```python
from build123d import *

# Parameters (mm, degrees)
SKETCH1_R               = 30
BOSS_EXTRUDE1_DEPTH     = 5
SKETCH2_R               = 20
SKETCH2_R_2             = 15
BOSS_EXTRUDE2_DEPTH     = 14.5
CUT_EXTRUDE1_START      = -20
SKETCH3_R               = 15
CUT_EXTRUDE1_DEPTH      = 20
CUT_EXTRUDE3_DEPTH      = 47.693147249
CUT_EXTRUDE3_DEPTH_BACK = 47.693147249
SKETCH5_R               = 2.5
SKETCH6_R               = 1.55
CUT_EXTRUDE4_DEPTH      = 10


with BuildPart() as part:
    # Sketch1 → Boss-Extrude1 (new body)
    with BuildSketch(Plane.XY):
        Circle(SKETCH1_R)
    extrude(amount=BOSS_EXTRUDE1_DEPTH)

    # Sketch2 → Boss-Extrude2 (add)
    with BuildSketch(Plane.XY.offset(5)):
        with Locations(Location((0, 0, 0), (0, 0, 180))):
            Circle(SKETCH2_R)
        with Locations(Location((0, 0, 0), (0, 0, 180))):
            Circle(SKETCH2_R_2, mode=Mode.SUBTRACT)
    extrude(amount=BOSS_EXTRUDE2_DEPTH)

    # Sketch3 → Cut-Extrude1 (cut)
    with BuildSketch(Plane.XY.offset(5).offset(CUT_EXTRUDE1_START)):
        with Locations(Location((0, 0, 0), (0, 0, 180))):
            Circle(SKETCH3_R)
    extrude(amount=CUT_EXTRUDE1_DEPTH, mode=Mode.SUBTRACT)

    # Sketch5 → Cut-Extrude3 (cut, two sides: drawn at the far end of the back side and taken through both)
    with BuildSketch(Plane(origin=(0, 0, 0), x_dir=(1, 0, 0), z_dir=(0, 1, 0)).offset(-CUT_EXTRUDE3_DEPTH_BACK)):
        with Locations(Location((0, -12.5, 0), (0, 0, 270))):
            Circle(SKETCH5_R)
    extrude(amount=CUT_EXTRUDE3_DEPTH + CUT_EXTRUDE3_DEPTH_BACK, mode=Mode.SUBTRACT)

    # Sketch6 → Cut-Extrude4 (cut)
    with BuildSketch(Plane.XY.offset(5)):
        with Locations((0, 25)):
            Circle(SKETCH6_R)
        with Locations((21.650635095, 12.5)):
            Circle(SKETCH6_R)
        with Locations((21.650635095, -12.5)):
            Circle(SKETCH6_R)
        with Locations((0, -25)):
            Circle(SKETCH6_R)
        with Locations((-21.650635095, -12.5)):
            Circle(SKETCH6_R)
        with Locations((-21.650635095, 12.5)):
            Circle(SKETCH6_R)
    extrude(amount=-CUT_EXTRUDE4_DEPTH, mode=Mode.SUBTRACT)


solid = part.part
```
Read the model definition and answer for the solid it produces. Units are mm, in the model's axes. A direction names the side the tool comes from. Coordinates: 2 decimals unless noted, no trailing zeros. Order: outer loops, then holes, each group sorted by start corner. A loop starts at its lowest first (then second) coordinate and runs counter-clockwise, first axis right, second up. Notation, with made-up numbers: (5.5, -11) - (48.5, -11) arc R18 cw to (48.5, -5) - close; hole circle Ø9 at (59, 2.25). An arc over 180 degrees is marked (long way). Answer as a JSON object with one key per item and string values. Group by question number.
Item 1: A tool of negligible diameter and unlimited length cuts with its end or side. For faces 1 (the face through (23.082, 11.906, 2.535)), 2 (the face through (20, 7, 5)), from which of +Z, -Z, +X, -X, +Y, -Y can it reach the whole face along a straight path? Write none if from no direction.
Item 2: Section A-A (y = 0) is taken. Give the vertices of the cut face in (x, z).
Item 3: The mould has two halves that part along Y. Classify faces 3 (the face through (0, 17, 10)), 4 (the face through (3.252, 14.643, 9.614)), 5 (the face through (19.98, -0.88, 12.15)): +Y half, -Y half, draft (parallel to the pull), parting line (faces both ways), or undercut.
Item 4: Section B-B (z = 4.25) is taken. Give the vertices of the cut face in (x, y).
Item 5: Section D-D (y = -12.5) is taken. Give the vertices of the cut face in (x, z), plus the area to 3 significant figures.
Item 6: Consider probe 1 along Y at (x, z) = (0, 1.9); probe 2 along Z at (x, y) = (0, -16.6); probe 3 along Y at (x, z) = (23, 1). Determine where each line is inside the solid, lowest interval first. Write a range as from..to.
Item 7: Section C-C (x = -13) is taken. Give the vertices of the cut face in (y, z), plus the area to 3 significant figures.
Item 8: Flat-ended cylindrical pins translate along their axes: P1, Ø10, axis at y = 10.5, z = 5, coming from the +X side; P2, Ø4, axis at x = -18.5, y = -23, coming from the +Z side; P3, Ø4, axis at y = 6.5, z = 14, coming from the +X side; P4, Ø3, axis at x = 0, z = 12.5, coming from the +Y side. Find the tip coordinate at first contact, or state that the pin passes through.
Results are:
{
 "1": {"face 1": "+Z, -Z", "face 2": "+Z"},
 "2": {"outline": "(-30, 0) - (-15, 0) - (-15, 19.5) - (-20, 19.5) - (-20, 5) - (-30, 5) - close; (15, 0) - (30, 0) - (30, 5) - (20, 5) - (20, 19.5) - (15, 19.5) - close"},
 "3": {"face 3": "draft", "face 4": "undercut", "face 5": "parting line"},
 "4": {"outline": "circle Ø60 at (0, 0); hole circle Ø3.1 at (-21.65, -12.5); hole circle Ø3.1 at (-21.65, 12.5); hole circle Ø30 at (0, 0); hole circle Ø3.1 at (0, -25); hole circle Ø3.1 at (0, 25); hole circle Ø3.1 at (21.65, -12.5); hole circle Ø3.1 at (21.65, 12.5)"},
 "5": {"outline": "(-27.27, 0) - (-23.2, 0) - (-23.2, 5) - (-27.27, 5) - close; (-20.1, 0) - (-8.29, 0) - (-8.29, 19.5) - (-15.61, 19.5) - (-15.61, 5) - (-20.1, 5) - close; (8.29, 0) - (20.1, 0) - (20.1, 5) - (15.61, 5) - (15.61, 19.5) - (8.29, 19.5) - close; (23.2, 0) - (27.27, 0) - (27.27, 5) - (23.2, 5) - close", "area": "371 mm^2"},
 "6": {"probe 1": "y = -30..-26.55, -23.45..-15, 15..23.45, 26.55..30", "probe 2": "z = 0..10, 15..19.5", "probe 3": "y = -19.26..-13.26, -11.74..11.74, 13.26..19.26"},
 "7": {"outline": "(-27.04, 0) - (-7.48, 0) - (-7.48, 19.5) - (-15.2, 19.5) - (-15.2, 5) - (-27.04, 5) - close; (7.48, 0) - (27.04, 0) - (27.04, 5) - (15.2, 5) - (15.2, 19.5) - (7.48, 19.5) - close", "area": "419 mm^2"},
 "8": {"P1": "stops at x = 29.49", "P2": "stops at z = 5", "P3": "stops at x = 19.49", "P4": "passes through"}
}
